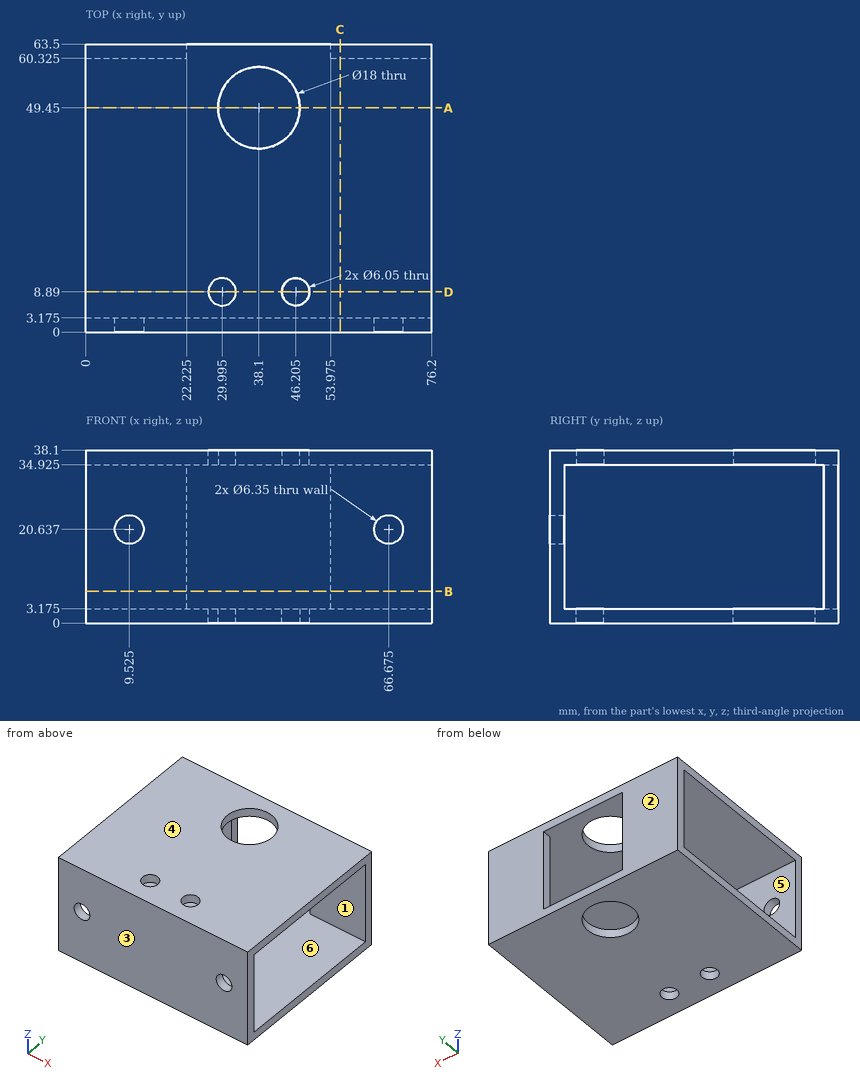
Geometry check sheet. Reference: drawing and pictorial views, mm from the part's lowest x, y, z. A direction names the side the tool comes from. Coordinates: 2 decimals unless noted, no trailing zeros. Order: outer loops, then holes, each group sorted by start corner. A loop starts at its lowest first (then second) coordinate and runs counter-clockwise, first axis right, second up. Notation, with made-up numbers: (28.25, 12.5) -> (45.25, 12.5) arc R33 cw to (45.25, 50.5) -> close; hole circle Ø10 at (61.25, -13). An arc over 180 degrees is marked (long way). Write item = value, one per line. Start each with the question number.
1) Cross-section at A-A (y = 49.45). Enter the section's corners in (x, z) (1 decimal).
2) Cross-section at B-B (z = 7). Enter the section's corners in (x, y) (1 decimal), then the cut area to 3 significant figures.
3) Material ranges on L1, parallel to Y at x = 38.1, z = 36; L2, parallel to Y at x = 54.5, z = 6 (1 decimal); L3, parallel to Z at x = 37.5, y = 28 (1 decimal), recorded low to high.
4) Cross-section at C-C (x = 56). Enter the section's corners in (y, z) (1 decimal).
5) Access from +Z, -Z, +X, -X, +Y, -Y to the whole of each face (thin tool, end or side, straight path). Record for the marked faces 1 and 2.
6) Go/stop test with flat-tipped pins: P1, Ø3.5, axis at x = 29.995, y = 8.89, coming from the +Z side; P2, Ø9.5, axis at x = 43.5, z = 22, coming from the +Y side (1 decimal). Record where each tip stops, or that it passes through.
7) Mould release check, pull along Z, two halves, no side actions. Record for the marked faces 3, 4, 5 and 6: +Z half, -Z half, draft (parallel to the pull), parting line (faces both ways), or undercut.
8) Cross-section at D-D (y = 8.89). Enter the section's corners in (x, z) (1 decimal).
Ans:
q1.outline = (0, 0) -> (29.1, 0) -> (29.1, 3.2) -> (0, 3.2) -> close; (0, 34.9) -> (29.1, 34.9) -> (29.1, 38.1) -> (0, 38.1) -> close; (47.1, 0) -> (76.2, 0) -> (76.2, 3.2) -> (47.1, 3.2) -> close; (47.1, 34.9) -> (76.2, 34.9) -> (76.2, 38.1) -> (47.1, 38.1) -> close
q2.outline = (0, 0) -> (76.2, 0) -> (76.2, 3.2) -> (0, 3.2) -> close; (0, 60.3) -> (22.2, 60.3) -> (22.2, 63.5) -> (0, 63.5) -> close; (54, 60.3) -> (76.2, 60.3) -> (76.2, 63.5) -> (54, 63.5) -> close
q2.area = 383 mm²
q3.L1 = 0 to 40.45, 58.45 to 63.5
q3.L2 = 0 to 3.2, 60.3 to 63.5
q3.L3 = 0 to 3.2, 34.9 to 38.1
q4.outline = (0, 0) -> (63.5, 0) -> (63.5, 38.1) -> (0, 38.1) -> close; hole (3.2, 3.2) -> (60.3, 3.2) -> (60.3, 34.9) -> (3.2, 34.9) -> close
q5.face_1 = +X, -X
q5.face_2 = +Z, -Z, +X, -X, +Y
q6.P1 = through
q6.P2 = 3.2
q7.face_3 = draft
q7.face_4 = +Z half
q7.face_5 = undercut
q7.face_6 = undercut
q8.outline = (0, 0) -> (27, 0) -> (27, 3.2) -> (0, 3.2) -> close; (0, 34.9) -> (27, 34.9) -> (27, 38.1) -> (0, 38.1) -> close; (33, 0) -> (43.2, 0) -> (43.2, 3.2) -> (33, 3.2) -> close; (33, 34.9) -> (43.2, 34.9) -> (43.2, 38.1) -> (33, 38.1) -> close; (49.2, 0) -> (76.2, 0) -> (76.2, 3.2) -> (49.2, 3.2) -> close; (49.2, 34.9) -> (76.2, 34.9) -> (76.2, 38.1) -> (49.2, 38.1) -> close
